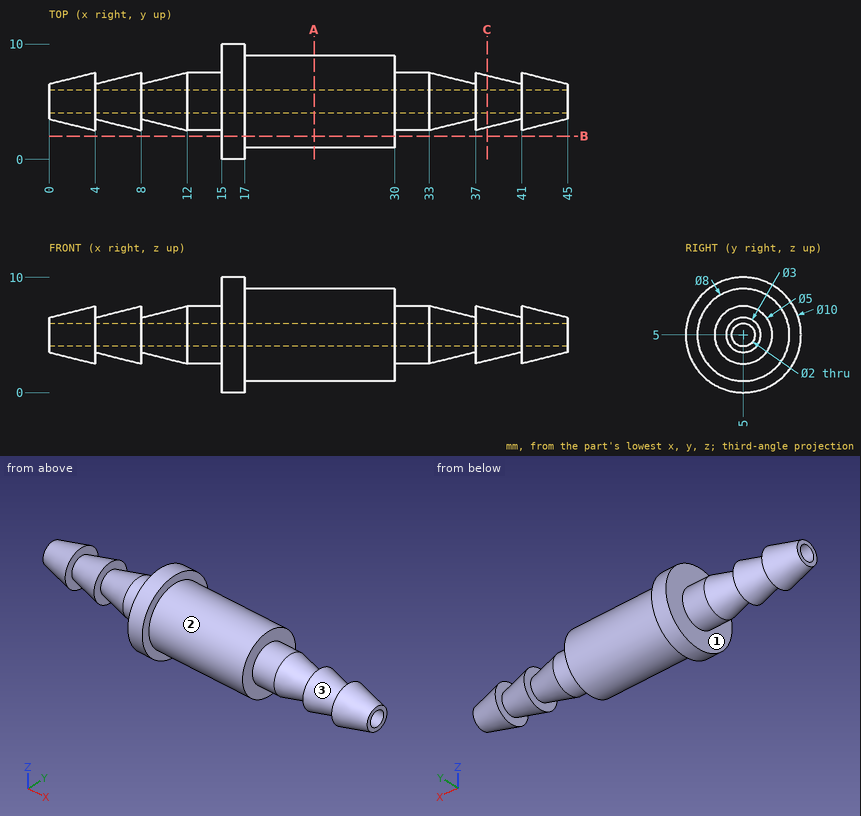
Study the drawing (mm; zero at the part's minimum x, y, z) and answer. A direction names the side the tool comes from. Give positions to 0.01 mm unless a question says otherwise; leave off trailing zeros. Write each loop counter-clockwise with the first axis right and the second up, starting at its lowest first coordinate (ties: lowest second). Pieces come first, ordered by that corner, then holes. Notation, with made-up numbers: (28.5, -7.75) -> (68.5, -7.75) arc R18 cw to (68.5, 7.25) -> close; hole circle Ø7 at (68, 72.25). An arc over 180 degrees is marked (long way). Answer in a Markdown table with one row per item.
1) Section B-B on y = 2 is taken. Give the vertices of the cut face in (x, z), plus the area to 3 significant figures.
Results list:
| item | result |
|---|---|
| outline | (15, 1) -> (17, 1) -> (17, 2.35) -> (30, 2.35) -> (30, 7.65) -> (17, 7.65) -> (17, 9) -> (15, 9) -> close |
| area | 84.8 mm^2 |
2) A tool of negligible diameter and unlimited length cuts with its end or side. For the marked faces 1, 2 and 3, from which of +Z, -Z, +X, -X, +Y, -Y can it reach the whole face along a straight path? Write none if from no direction.
Results list:
| item | result |
|---|---|
| face 1 | -X |
| face 2 | +X |
| face 3 | none |
3) Section A-A on x = 23 is taken. Give the vertices of the cut face in (y, z).
Results list:
| item | result |
|---|---|
| outline | circle Ø8 at (5, 5); hole circle Ø2 at (5, 5) |
4) Section C-C on x = 38 is taken. Give the vertices of the cut face in (y, z), plus the area to 3 significant figures.
Results list:
| item | result |
|---|---|
| outline | circle Ø4.5 at (5, 5); hole circle Ø2 at (5, 5) |
| area | 12.8 mm^2 |
5) Straight lines are drawn through the part: line 1 (X direction, y = 5.5, z = 2.25); line 2 (X direction, y = 0.75, z = 5.75); line 3 (Y direction, x = 9, z = 5). For each, find the intervals that lie inside material, in ascending order. Write a range as [from, to].
Results list:
| item | result |
|---|---|
| line 1 | [15, 30] |
| line 2 | [15, 17] |
| line 3 | [3.25, 4], [6, 6.75] |
6) Each of these flat-tipped pins is pushed along its axis until it touches: pin 1 Ø3 at (x, y) = (29.5, 4.5) entering from +Z; pin 2 Ø1 at (y, z) = (4.5, 3.5) entering from -X; pin 3 Ø1.2 at (y, z) = (5, 5) entering from -X; pin 4 Ø1.5 at (x, y) = (37.5, 6.5) entering from +Z. Where does it stop, or does it pass through?
Results list:
| item | result |
|---|---|
| pin 1 | z = 9 |
| pin 2 | x = 0 |
| pin 3 | through |
| pin 4 | z = 7.32 |
